Read the model definition and answer for the solid it produces. Units are mm, in the model's axes. Give positions to 0.01 mm unless a question says otherwise; leave off trailing zeros. Answer as CSV lines item,"result". Start each with the question number.
from build123d import *

# Parameters (mm, degrees)
BOSS_EXTRUDE1_DEPTH = 650
BOSS_EXTRUDE2_START = -0.7112
BOSS_EXTRUDE2_DEPTH = 0.7112
LPATTERN1_COUNT     = 11
LPATTERN1_PITCH     = 64.929


# Read off the part's stored shape, not the designer's step: Boss-Extrude2
with BuildPart() as part:
    # Sketch1 → Boss-Extrude1 (new body)
    with BuildSketch(Plane.XY):
        with BuildLine():
            add(Edge.make_bspline(
                [(-112.898494578, 0.99146631), (-110.355982987, 1.262339099), (-105.259380368, 1.808389528), (-95.162712882, 2.902575782), (-82.658600361, 4.281227817), (-67.864804262, 5.950995414), (-48.419089864, 8.198779354), (-24.648701462, 11.048580313), (2.987237789, 14.533371756), (29.350050206, 18.036965667), (47.273220771, 20.55034649), (57.461014612, 22.023800415), (59.555137323, 22.328856294), (60.599627559, 22.481560095)],
                knots=[0.938155776, 0.938155776, 0.938155776, 0.938155776, 0.940088408, 0.94202104, 0.945886304, 0.949751568, 0.953616832, 0.96134736, 0.969077888, 0.976808416, 0.984232202, 0.985198518, 0.986164834, 0.986164834, 0.986164834, 0.986164834], degree=3))
            Line((60.599627559, 22.481560095), (104.654430058, 24.21413648))
            add(Edge.make_bspline(
                [(-112.368804727, -3.980397391), (-30.684146875, 4.722080559), (42.524377626, 14.095206887), (104.654430058, 24.21413648)],
                knots=[0.938155776, 0.938155776, 0.938155776, 0.938155776, 1, 1, 1, 1], degree=3))
            Line((-112.368804727, -3.980397391), (-112.898494578, 0.99146631))
        make_face()
    extrude(amount=BOSS_EXTRUDE1_DEPTH)

    # Boss-Extrude2 outline → Boss-Extrude2 (add)
    with BuildSketch(Plane.XY.offset(650).offset(BOSS_EXTRUDE2_START)):
        with BuildLine():
            ThreePointArc((-82.963014518, 68.430375082), (-105.947446125, 64.342164511), (-115.534774611, 43.056472263))
            Line((-115.534774611, 43.056472263), (-112.898494578, 0.99146631))
            add(Edge.make_bspline(
                [(-112.898494578, 0.99146631), (-110.355982987, 1.262339099), (-105.259380368, 1.808389528), (-95.162712882, 2.902575782), (-82.658600361, 4.281227817), (-67.864804262, 5.950995414), (-48.419089864, 8.198779354), (-24.648701462, 11.048580313), (2.987237789, 14.533371756), (29.350050206, 18.036965667), (47.273220771, 20.55034649), (57.461014612, 22.023800415), (59.555137323, 22.328856294), (60.599627559, 22.481560095)],
                knots=[0.938155776, 0.938155776, 0.938155776, 0.938155776, 0.940088408, 0.94202104, 0.945886304, 0.949751568, 0.953616832, 0.96134736, 0.969077888, 0.976808416, 0.984232202, 0.985198518, 0.986164834, 0.986164834, 0.986164834, 0.986164834], degree=3))
            Line((60.599627559, 22.481560095), (-82.963014518, 68.430375082))
        make_face()
    boss_extrude2 = extrude(amount=BOSS_EXTRUDE2_DEPTH)

    # LPattern1: Boss-Extrude2 ×11
    with Locations(*[(0, 0, -i * LPATTERN1_PITCH) for i in range(1, LPATTERN1_COUNT)]):
        add(boss_extrude2)


solid = part.part
(1) Flat-ended cylindrical pins translate along their axes: pin 1 Ø20.5 at (x, y) = (0, 46.5) entering from -Z; pin 2 Ø4 at (x, z) = (-0.5, 318.5) entering from -Y; pin 3 Ø1.5 at (x, z) = (-2.5, 258.5) entering from -Y; pin 4 Ø12 at (x, z) = (-40, 289) entering from +Y. Find the tip coordinate at first contact, or state that the pin passes through.
(2) Determine the mould class of faces 1 (the flat face through (-56, 33, 650)), 2 (the cylindrical face through (-105.68, 64.55, 130.21)), 3 (the flat face through (-48, 36, 649.289)) for opening direction Z: released by +Z, released by -Z, zero draft, split by the parting line, or undercut.
(3) Straight lines are drawn through the part: line 1 (Y direction, x = -99.5, z = 64.5); line 2 (Y direction, x = -98, z = 548.5). For each, find the intervals that lie inside material, in ascending order. Write a range as [from, to].
(4) Section A-A, the plane y = 58.5 is taken. State how many separate pieces and enclosed holes the cut face has, and give its area (3 significant figures).
Checks:
1,pin 1,"stops at z = 0"
1,pin 2,"stops at y = 8.82"
1,pin 3,"stops at y = 8.72"
1,pin 4,"stops at y = 9.94"
2,face 1,"released by +Z"
2,face 2,"zero draft"
2,face 3,"undercut"
3,line 1,"y = [-2.6, 2.43]"
3,line 2,"y = [-2.43, 2.6]"
4,separate pieces,"11"
4,enclosed holes,"0"
4,area,"465 mm²"
